Input: part model. Units: mm. Frame: model coordinates. Coordinates: 2 decimals unless noted, no trailing zeros. Loops run counter-clockwise (first coordinate to the right, second up) from the corner with the lowest first, then second, coordinate; pieces in that order, holes last.
Item 1: Ray query, line 1 along X through (y, z) = (133, 0.55); line 2 along Y through (x, z) = (100, 1.15); line 3 along X through (y, z) = (107, 0.65). Return the intervals inside material, ascending.
Item 2: Section A-A on z = 0.5. Give the number of separate pieces and of enclosed holes in the cut face, and give its area (3 significant figures).
Item 3: Contact query for a flat-ended pin moving along its axis: P1, Ø8, axis at x = 63.14, y = 35, coming from the +Z side. Output: stop coordinate, or through.
Item 4: Section C-C on y = 145. Return loops of the section in (x, z), and give its area (3 significant figures).
Item 5: Section D-D on y = 15. Return loops of the section in (x, z).
Item 6: Section B-B on y = 70. Return loops of the section in (x, z).
```python
from build123d import *

# Parameters (mm, degrees)
SKETCH1_R           = 4.5
SKETCH1_R_2         = 2
BOSS_EXTRUDE1_DEPTH = 2
FILLET1_R           = 30
FILLET2_R           = 10


with BuildPart() as part:
    # Sketch1 → Boss-Extrude1 (new body)
    with BuildSketch(Plane.XY):
        Polygon((0, 0), (98.729357602, 158), (293.729357602, 158), (357.565501284, 0), align=None)
        with Locations((284.960746883, 145)):
            Circle(SKETCH1_R, mode=Mode.SUBTRACT)
        with Locations((305.675867386, 35)):
            Circle(SKETCH1_R, mode=Mode.SUBTRACT)
        with Locations((63.141671434, 35)):
            Circle(SKETCH1_R, mode=Mode.SUBTRACT)
        with Locations((163.141671434, 15)):
            Circle(SKETCH1_R, mode=Mode.SUBTRACT)
        with Locations((228.729357602, 70)):
            Circle(SKETCH1_R, mode=Mode.SUBTRACT)
        with Locations((100, 128)):
            Circle(SKETCH1_R, mode=Mode.SUBTRACT)
        with Locations((243.729357602, 133)):
            Circle(SKETCH1_R_2, mode=Mode.SUBTRACT)
        with Locations((143.729357602, 133)):
            Circle(SKETCH1_R_2, mode=Mode.SUBTRACT)
        with Locations((297.565501284, 128)):
            Circle(SKETCH1_R_2, mode=Mode.SUBTRACT)
        with Locations((287.565501284, 128)):
            Circle(SKETCH1_R_2, mode=Mode.SUBTRACT)
        with BuildLine():
            Line((105.935375271, 149.5), (123.935375271, 149.5))
            ThreePointArc((123.935375271, 149.5), (128.435375271, 145), (123.935375271, 140.5))
            Line((123.935375271, 140.5), (105.935375271, 140.5))
            ThreePointArc((105.935375271, 140.5), (101.435375271, 145), (105.935375271, 149.5))
        make_face(mode=Mode.SUBTRACT)
    extrude(amount=BOSS_EXTRUDE1_DEPTH)

    # Fillet1
    fillet1_edges = [part.edges().sort_by_distance(p)[0] for p in [
        (0, 0, 1),
        (357.565501284, 0, 1),
    ]]
    fillet(fillet1_edges, radius=FILLET1_R)

    # Fillet2
    fillet2_edges = [part.edges().sort_by_distance(p)[0] for p in [
        (98.729357602, 158, 1),
        (293.729357602, 158, 1),
    ]]
    fillet(fillet2_edges, radius=FILLET2_R)


solid = part.part
```
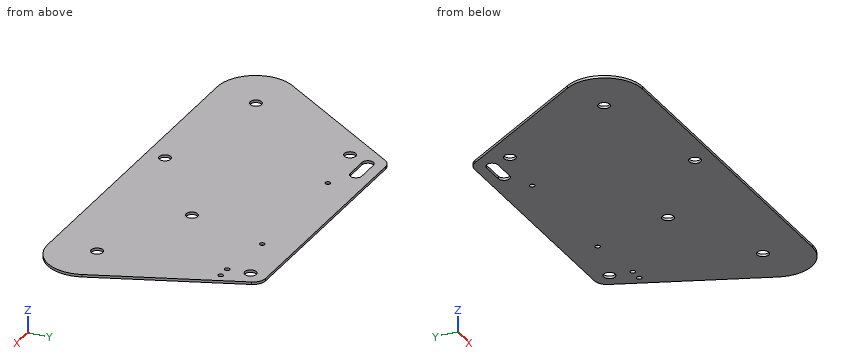
Results found:
1. line 1: x = 83.11 to 141.73, 145.73 to 241.73, 245.73 to 303.83
1. line 2: y = 0 to 123.5, 132.5 to 157.04
1. line 3: x = 66.86 to 314.33
2. separate pieces: 1
2. enclosed holes: 11
2. area: 41,900 mm2
3. P1: passes through
4. outline: (90.61, 0) - (101.44, 0) - (101.44, 2) - (90.61, 2) - close; (128.44, 0) - (280.46, 0) - (280.46, 2) - (128.44, 2) - close; (289.46, 0) - (298.98, 0) - (298.98, 2) - (289.46, 2) - close
4. area: 345 mm2
5. outline: (28.14, 0) - (158.64, 0) - (158.64, 2) - (28.14, 2) - close; (167.64, 0) - (339.07, 0) - (339.07, 2) - (167.64, 2) - close
6. outline: (43.74, 0) - (224.23, 0) - (224.23, 2) - (43.74, 2) - close; (233.23, 0) - (329.28, 0) - (329.28, 2) - (233.23, 2) - close
